from build123d import *

# Parameters (mm, degrees)
BOSS_EXTRUDE1_DEPTH = 1.27
SKETCH2_R           = 2.413
CUT_EXTRUDE1_DEPTH  = 58.557767504
LPATTERN1_COUNT     = 5
LPATTERN1_PITCH     = 25.4


with BuildPart() as part:
    # Sketch1 → Boss-Extrude1 (new, symmetric)
    with BuildSketch(Plane.XY):
        with BuildLine():
            Line((-50.8, 6.35), (50.8, 6.35))
            ThreePointArc((50.8, 6.35), (57.15, 0), (50.8, -6.35))
            Line((50.8, -6.35), (-50.8, -6.35))
            ThreePointArc((-50.8, -6.35), (-57.15, 0), (-50.8, 6.35))
        make_face()
    extrude(amount=BOSS_EXTRUDE1_DEPTH, both=True)

    # Sketch2 → Cut-Extrude1 (cut, through all)
    with BuildSketch(Plane.XY.offset(1.27)):
        with Locations((-50.8, 0)):
            Circle(SKETCH2_R)
    cut_extrude1 = extrude(amount=-CUT_EXTRUDE1_DEPTH, mode=Mode.SUBTRACT)

    # LPattern1: Cut-Extrude1 ×5
    with Locations(*[(i * LPATTERN1_PITCH, 0, 0) for i in range(1, LPATTERN1_COUNT)]):
        add(cut_extrude1, mode=Mode.SUBTRACT)


solid = part.part
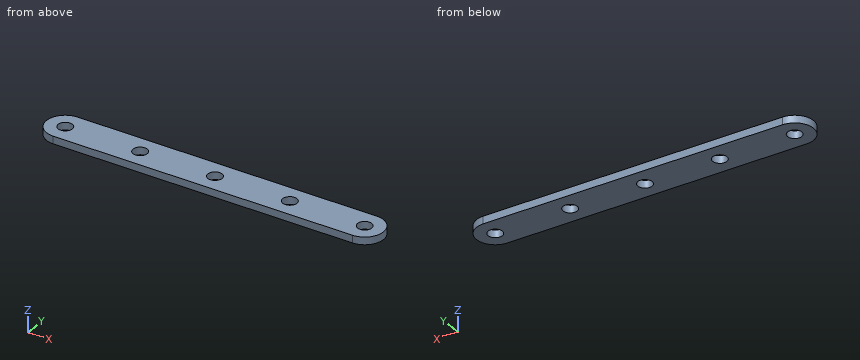
The listing builds one solid part. Answer for the finished solid, in the listing's coordinates (mm). Coordinates: 2 decimals unless noted, no trailing zeros. Write each loop counter-clockwise with the first axis right and the second up, starting at its lowest first coordinate (ties: lowest second). Pieces come first, ordered by that corner, then holes. Notation, with made-up numbers: M 44,68 L 81,68 A29 cw 81,107 Z; hole C 10,34 d10. An arc over 180 degrees is marked long. Write each question's results on one line, items separated by ' | '.
Item 1: Consider probe 1 along X at (y, z) = (-0.5, -0.9); probe 2 along Y at (x, z) = (0, -0.5); probe 3 along X at (y, z) = (0.75, -0.25). Determine where each line is inside the solid, lowest interval first. Write a range as [from, to].
Answer below:
probe 1: [-57.13, -53.16], [-48.44, -27.76], [-23.04, -2.36], [2.36, 23.04], [27.76, 48.44], [53.16, 57.13] | probe 2: [-6.35, -2.41], [2.41, 6.35] | probe 3: [-57.11, -53.09], [-48.51, -27.69], [-23.11, -2.29], [2.29, 23.11], [27.69, 48.51], [53.09, 57.11]
Item 2: The part is cut by section A-A on z = -0.1. Determine the outline of the cut face in (x, y), and give its area (3 significant figures).
Answer below:
outline: M -50.8,-6.35 L 50.8,-6.35 A6.35 ccw 50.8,6.35 L -50.8,6.35 A6.35 ccw Z; hole C -50.8,0 d4.83; hole C -25.4,0 d4.83; hole C 0,0 d4.83; hole C 25.4,0 d4.83; hole C 50.8,0 d4.83 | area: 1,330 mm2
Item 3: The part is cut by section B-B on x = -25.4. Determine the outline of the cut face in (y, z).
Answer below:
outline: M -6.35,-1.27 L -2.41,-1.27 L -2.41,1.27 L -6.35,1.27 Z; M 2.41,-1.27 L 6.35,-1.27 L 6.35,1.27 L 2.41,1.27 Z
Item 4: The part is cut by section C-C on y = -4.5. Determine the outline of the cut face in (x, z), and give its area (3 significant figures).
Answer below:
outline: M -55.28,-1.27 L 55.28,-1.27 L 55.28,1.27 L -55.28,1.27 Z | area: 281 mm2
